The model under review builds one solid part; all positions refer to its coordinate system, in mm. Face numbers are marked on the shaded views. A direction names the side the tool comes from. Give positions to 0.01 mm unless a question says otherwise; leave off trailing zeros. Loops run counter-clockwise (first coordinate to the right, second up) from the corner with the lowest first, then second, coordinate; pieces in that order, holes last. Notation, with made-up numbers: M 12.5,88.5 L 70.5,88.5 A19 cw 70.5,114.5 Z; hole C 4.5,9 d5. An arc over 180 degrees is marked long. Put each result on its own line as item: value. Start each with the question number.
from build123d import *

# Parameters (mm, degrees)
SKETCH1_W                    = 125
SKETCH1_H                    = 73.5
BASE_FLANGE1_DEPTH           = 2.1
EDGE_FLANGE1_STRIP_W         = 12.6
EDGE_FLANGE1_STRIP_H         = 2.1
EDGE_FLANGE1_STRIP_CUT_DEPTH = 125
EDGE_FLANGE1_DEPTH           = 125
CUT_EXTRUDE1_REACH           = 148.302
PSU_MOUNTING_HOLES_D         = 3.6576
FILLET1_R                    = 1
SSD_MOUNTING_HOLES_D         = 3.4
M3_CLEARANCE_HOLE1_D         = 3.4
EDGE_FLANGE2_DEPTH           = 58.5
EDGE_FLANGE2_BEND_DEPTH      = 58.5
FILLET2_R                    = 4


# Sheet-metal steps are written as plain solids
with BuildPart() as part:
    # Sketch1 → Base-Flange1 (new body)
    with BuildSketch(Plane(origin=(0, 0, 0), x_dir=(1, 0, 0), z_dir=(0, 1, 0))):
        with Locations((62.5, 36.75)):
            Rectangle(SKETCH1_W, SKETCH1_H)
    extrude(amount=-BASE_FLANGE1_DEPTH)

    # Edge-Flange1 strip (across the edge) → Edge-Flange1 strip cut (cut)
    with BuildSketch(Plane(origin=(0, -2.1, -73.5), x_dir=(0, 0, 1), z_dir=(1, 0, 0))):
        with Locations((-4.2, -1.05)):
            Rectangle(EDGE_FLANGE1_STRIP_W, EDGE_FLANGE1_STRIP_H)
    extrude(amount=EDGE_FLANGE1_STRIP_CUT_DEPTH, mode=Mode.SUBTRACT)

    # Edge-Flange1 section (across the edge) → Edge-Flange1 (add)
    with BuildSketch(Plane(origin=(0, -2.1, -73.5), x_dir=(0, 0, 1), z_dir=(1, 0, 0))):
        with BuildLine():
            Line((-2.1, 2.1), (-2.1, 8))
            Line((-2.1, 8), (0, 8))
            Line((0, 8), (0, 2.1))
            ThreePointArc((0, 2.1), (0.61507576, 0.61507576), (2.1, 0))
            Line((2.1, 0), (2.1, -2.1))
            ThreePointArc((2.1, -2.1), (-0.869848481, -0.869848481), (-2.1, 2.1))
        make_face()
    extrude(amount=EDGE_FLANGE1_DEPTH)

    # Sketch7 → Cut-Extrude1 (cut, up to next)
    with BuildSketch(Plane(origin=(0, -2.1, 0), x_dir=(-1, 0, 0), z_dir=(0, -1, 0)), mode=Mode.PRIVATE) as cut_extrude1_sk1:
        Polygon((-115.625, 28.375), (-119, 28.375), (-119, 9.375), (-115.625, 9.375), (-115.625, 4.3), (-9.375, 4.3), (-9.375, 9.375), (-6, 9.375), (-6, 28.375), (-9.375, 28.375), (-9.375, 35.125), (-6, 35.125), (-6, 54.125), (-9.375, 54.125), (-9.375, 63.5), (-115.625, 63.5), (-115.625, 54.125), (-119, 54.125), (-119, 35.125), (-115.625, 35.125), align=None)
    cut_extrude1_tool1 = extrude(cut_extrude1_sk1.sketch, amount=-CUT_EXTRUDE1_REACH, mode=Mode.PRIVATE) & part.part
    add(cut_extrude1_tool1.solids().sort_by_distance((62.5, -2.1, -33.81576))[0], mode=Mode.SUBTRACT)

    # psu-mounting-holes (through all)
    with Locations(Plane(origin=(0, 0, 0), x_dir=(1, 0, 0), z_dir=(0, 1, 0))):
        with Locations((119, 6), (119, 57.5), (6, 6), (6, 57.5), (6, 31.75), (119, 31.75)):
            Hole(PSU_MOUNTING_HOLES_D / 2)

    # Fillet1
    fillet1_edges = [part.edges().sort_by_distance(p)[0] for p in [
        (119, -1.05, -28.375),
        (115.625, -1.05, -28.375),
        (115.625, -1.05, -35.125),
        (119, -1.05, -35.125),
        (119, -1.05, -54.125),
        (115.625, -1.05, -54.125),
        (115.625, -1.05, -63.5),
        (9.375, -1.05, -63.5),
        (9.375, -1.05, -54.125),
        (6, -1.05, -54.125),
        (6, -1.05, -35.125),
        (9.375, -1.05, -35.125),
        (9.375, -1.05, -28.375),
        (6, -1.05, -28.375),
        (6, -1.05, -9.375),
        (9.375, -1.05, -9.375),
        (9.375, -1.05, -4.3),
        (115.625, -1.05, -4.3),
        (115.625, -1.05, -9.375),
        (119, -1.05, -9.375),
    ]]
    fillet(fillet1_edges, radius=FILLET1_R)

    # ssd-mounting-holes (through all)
    with Locations(Plane(origin=(0, 0, 0), x_dir=(1, 0, 0), z_dir=(0, 1, 0))):
        with Locations((115.1, 67.5), (38.5, 67.5)):
            Hole(SSD_MOUNTING_HOLES_D / 2)

    # M3 Clearance Hole1 (through all)
    with Locations(Plane.XY.offset(-73.5)):
        with Locations((120, -7.15), (5, -7.15)):
            Hole(M3_CLEARANCE_HOLE1_D / 2)

    # Edge-Flange2 section (across the edge) → Edge-Flange2 (add)
    with BuildSketch(Plane(origin=(127.1, 0, -5), x_dir=(-1, 0, 0), z_dir=(0, 0, -1))):
        with BuildLine():
            Line((-2.1, 2.1), (-2.1, 7.9))
            Line((-2.1, 7.9), (0, 7.9))
            Line((0, 7.9), (0, 2.1))
            ThreePointArc((0, 2.1), (0.61507576, 0.61507576), (2.1, 0))
            Line((2.1, 0), (2.1, -2.1))
            ThreePointArc((2.1, -2.1), (-0.869848481, -0.869848481), (-2.1, 2.1))
        make_face()
    extrude(amount=EDGE_FLANGE2_DEPTH)

    # Edge-Flange2 section 2 (across the edge) → Edge-Flange2 bend (add)
    with BuildSketch(Plane(origin=(-2.1, 0, -63.5), x_dir=(1, 0, 0), z_dir=(0, 0, 1))):
        with BuildLine():
            Line((-2.1, 2.1), (-2.1, 7.9))
            Line((-2.1, 7.9), (0, 7.9))
            Line((0, 7.9), (0, 2.1))
            ThreePointArc((0, 2.1), (0.61507576, 0.61507576), (2.1, 0))
            Line((2.1, 0), (2.1, -2.1))
            ThreePointArc((2.1, -2.1), (-0.869848481, -0.869848481), (-2.1, 2.1))
        make_face()
    extrude(amount=EDGE_FLANGE2_BEND_DEPTH)

    # Fillet2
    fillet2_edges = [part.edges().sort_by_distance(p)[0] for p in [
        (128.15, 7.9, -5),
        (128.15, 7.9, -63.5),
        (0, -10.1, -74.55),
        (-3.15, 7.9, -63.5),
        (-3.15, 7.9, -5),
        (125, -10.1, -74.55),
        (125, -1.05, 0),
        (0, -1.05, 0),
    ]]
    fillet(fillet2_edges, radius=FILLET2_R)


solid = part.part
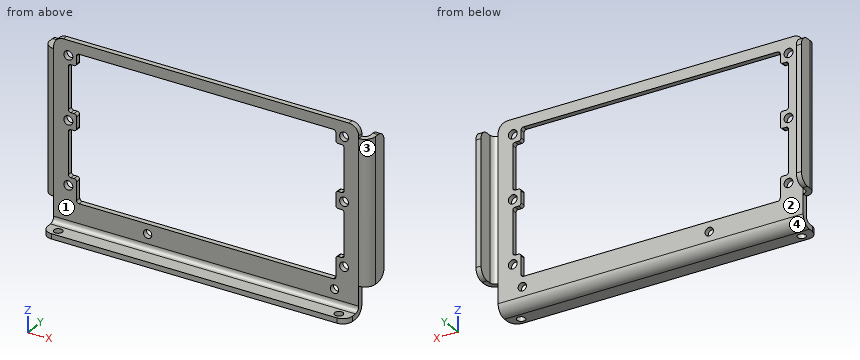
(1) Insertion check: pin 1 (12 mm diameter, centred on x = 115.5, z = -49.5, fed in from +Y); pin 2 (2.5 mm diameter, centred on y = -1.5, z = -59.5, fed in from +X); pin 3 (4.5 mm diameter, centred on x = 127.5, y = 1, fed in from -Z). Each pin has a flat end and moves straight along its axis. Give the tip position at first contact, or say it passes through.
(2) We need section A-A, the plane x = 110. Write out the cut boundary in (y, z), plus the area to 3 significant figures.
(3) To check wall thickness, follow L1, parallel to X at y = 6.5, z = -42; L2, parallel to Z at x = 72.5, y = -6; L3, parallel to X at y = -1.5, z = -23.5. State the ranges of each line that lie inside material, in increasing order. Write a range as [from, to].
(4) We need section C-C, the plane y = 5.75. Write out the cut boundary in (x, z), plus the area to 3 significant figures.
(5) For the marked faces 1 and 2, list the 3-axis set-ups (+Z, -Z, +X, -X, +Y, -Y) from which the entire face can be reached by the end or side of a thin tool; tool diameter is ignored.
(6) We need section B-B, the plane z = -57.5. Write out the cut boundary in (x, y) (3 decimals).
(7) Draft analysis for pull direction Y (two halves, no side actions). For the marked faces 3 and 4, state which applies: +Y half, -Y half, draft (parallel to the pull), parting line (faces both ways), or undercut.
Check sheet entries:
1. pin 1: stops at y = 0
1. pin 2: stops at x = 128.48
1. pin 3: stops at z = -63.5
2. outline: M -10.1,-75.6 L -4.2,-75.6 A4.2 ccw 0,-71.4 L 0,-63.5 L -2.1,-63.5 L -2.1,-71.4 A2.1 cw -4.2,-73.5 L -10.1,-73.5 Z; M -2.1,-4.3 L 0,-4.3 L 0,0 L -2.1,0 Z
2. area: 48.4 mm²
3. L1: x = [-4.2, -2.1], [127.1, 129.2]
3. L2: z = [-75.6, -73.5]
3. L3: x = [-2.16, 6], [119, 127.16]
4. outline: M -4.2,-63.05 L -2.1,-63.05 L -2.1,-5.45 L -4.2,-5.45 Z; M 127.1,-63.05 L 129.2,-63.05 L 129.2,-5.45 L 127.1,-5.45 Z
4. area: 242 mm²
5. face 1: +Z, +X, -X, -Y
5. face 2: +Z, -Z, +Y
6. outline: M -4.2,2.1 A4.2 ccw 0,-2.1 L 4.171,-2.1 L 4.171,0 L 0,0 A2.1 cw -2.1,2.1 L -2.1,7.9 L -4.2,7.9 Z; M 7.829,-2.1 L 9.375,-2.1 L 9.375,0 L 7.829,0 Z; M 115.625,-2.1 L 117.171,-2.1 L 117.171,0 L 115.625,0 Z; M 120.829,-2.1 L 125,-2.1 A4.2 ccw 129.2,2.1 L 129.2,7.9 L 127.1,7.9 L 127.1,2.1 A2.1 cw 125,0 L 120.829,0 Z
7. face 3: -Y half
7. face 4: +Y half
